from build123d import *

# Parameters (mm, degrees)
F0_R     = 12.5
F0_R_2   = 6.5
F0_R_3   = 4.5
F1_DEPTH = 2
F2_DEPTH = 10
F3_SIZE  = 1.8


with BuildPart() as f1:
    # F0 (on Top) → F1 (new body)
    with BuildSketch(Plane.XY):
        Circle(F0_R)
        Circle(F0_R_2, mode=Mode.SUBTRACT)
        Circle(F0_R_2)
        Circle(F0_R_3, mode=Mode.SUBTRACT)
        Circle(F0_R_3)
    extrude(amount=F1_DEPTH)

    # F0 (on Top) → F2 (join)
    with BuildSketch(Plane.XY):
        Circle(F0_R_2)
        Circle(F0_R_3, mode=Mode.SUBTRACT)
    extrude(amount=F2_DEPTH)

    # F3
    f3_edges = [f1.edges().sort_by_distance(p)[0] for p in [
        (-12.5, 0, 0),
    ]]
    chamfer(f3_edges, length=F3_SIZE)


solid = f1.part
Build history of the part. All positions in model axes, mm. A direction names the side the tool comes from. Coordinates: 2 decimals unless noted, no trailing zeros. Order: outer loops, then holes, each group sorted by start corner. A loop starts at its lowest first (then second) coordinate and runs counter-clockwise, first axis right, second up. Notation, with made-up numbers: (39, 69) - (84, 69) arc R17 cw to (84, 76) - close; hole circle Ø1 at (56, 44.25). An arc over 180 degrees is marked (long way). Write each question's results on one line, items separated by ' | '. Start each with the question number.
Item 1: Flat gauge pins, fed straight in: pin 1 (6 mm diameter, centred on y = 8, z = 8, fed in from +X); pin 2 (8 mm diameter, centred on x = -9.5, y = 10, fed in from +Z); pin 3 (4 mm diameter, centred on y = -6, z = 2, fed in from -X). Where does each tip first touch, or does it go through?
Item 2: Tool access for faces 1 (the face through (-4.42, 1.54, 10)), 2 (the face through (-0.59, 4.46, 5.94)): list every direction of +Z, -Z, +X, -X, +Y, -Y with a clear straight run to the whole face (end or side of a thin tool).
Item 3: Band-saw the part on A-A on x = 0. Write the cut outline in (y, z), and give its area (3 significant figures).
Item 4: Band-saw the part on D-D on z = 1. Write the cut outline in (x, y), and give its area (3 significant figures).
Item 5: Wall check: probe 1 along Y at (x, z) = (0, 7.25); probe 2 along Z at (x, y) = (-7.25, -2). Give the ranges that are in metal, low to high. Write a range as [from, to].
Item 6: Band-saw the part on B-B on z = 6.75. Write the cut outline in (x, y), and give its area (3 significant figures).
Item 7: Mould opens along X. For faces 3 (the face through (0, 0, 2)), 4 (the face through (-2.344, -10.555, 0.113)), 5 (the face through (0, 0, 0)) say: released by +X, released by -X, zero draft, split by the parting line, or undercut.
Numbers:
1) pin 1: x = 4.15 | pin 2: z = 2 | pin 3: x = -11.84
2) face 1: +Z, +X, -X, +Y, -Y | face 2: +Z
3) outline: (-12.5, 1.8) - (-10.7, 0) - (10.7, 0) - (12.5, 1.8) - (12.5, 2) - (6.5, 2) - (6.5, 10) - (4.5, 10) - (4.5, 2) - (-4.5, 2) - (-4.5, 10) - (-6.5, 10) - (-6.5, 2) - (-12.5, 2) - close | area: 78.8 mm^2
4) outline: circle Ø23.4 at (0, 0) | area: 430 mm^2
5) probe 1: [-6.5, -4.5], [4.5, 6.5] | probe 2: [0, 2]
6) outline: circle Ø13 at (0, 0); hole circle Ø9 at (0, 0) | area: 69.1 mm^2
7) face 3: undercut | face 4: split by the parting line | face 5: zero draft
